Check sheet for the modelled part. Datum: model origin and axes. Units: mm. Face numbers are marked on the shaded views. A direction names the side the tool comes from. Give positions to 0.01 mm unless a question says otherwise; leave off trailing zeros. Order: outer loops, then holes, each group sorted by start corner. A loop starts at its lowest first (then second) coordinate and runs counter-clockwise, first axis right, second up.
from build123d import *

# Parameters (mm, degrees)
SKETCH2_R           = 6.5
BOSS_EXTRUDE1_DEPTH = 7


with BuildPart() as part:
    # Sketch1 → Revolve1 (revolve)
    with BuildSketch(Plane.XY):
        with BuildLine():
            Line((0, 6.5), (0, 10.5))
            Line((0, 10.5), (22.5, 10.5))
            Line((22.5, 10.5), (22.5, 7.5))
            Line((22.5, 7.5), (10.5, 7.5))
            ThreePointArc((10.5, 7.5), (10.146446609, 7.353553391), (10, 7))
            Line((10, 7), (10, 6.5))
            Line((10, 6.5), (0, 6.5))
        make_face()
    revolve(axis=Axis((0, 0, 0), (1, 0, 0)))

    # Sketch2 → Boss-Extrude1 (add)
    with BuildSketch(Plane.ZY):
        Polygon((0, 13.279056191), (-11.5, 6.639528096), (-11.5, -6.639528096), (0, -13.279056191), (11.5, -6.639528096), (11.5, 6.639528096), align=None)
        Circle(SKETCH2_R, mode=Mode.SUBTRACT)
    extrude(amount=-BOSS_EXTRUDE1_DEPTH)

    # Cut-Sweep1: sweep along a path in Sketch6
    with BuildLine(Plane.ZY) as cut_sweep1_path:
        CenterArc((0, 0), 11.5, 0, 360)
    # Sketch5 → Cut-Sweep1 (sweep, cut)
    with BuildSketch(Plane.XY):
        with BuildLine():
            Line((0.6, 13.279056191), (0, 13.279056191))
            Line((0, 13.279056191), (0, 11))
            ThreePointArc((0, 11), (0.152512755, 12.178356602), (0.6, 13.279056191))
        make_face()
    sweep(path=cut_sweep1_path.line, mode=Mode.SUBTRACT)


solid = part.part
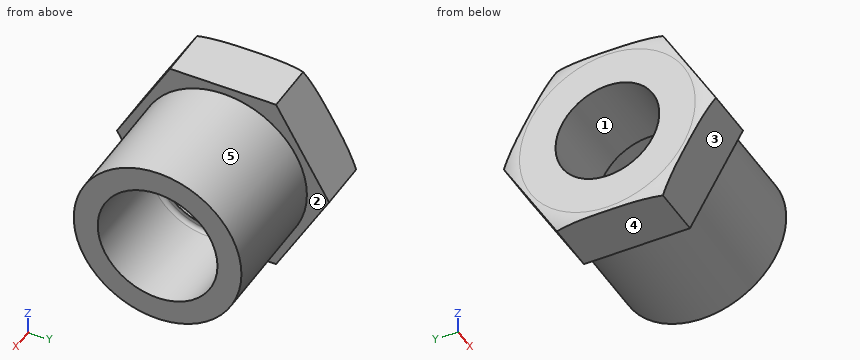
1) Set-up check for the marked faces 4 and 5: record each of +Z, -Z, +X, -X, +Y, -Y from which the full face is reachable in a straight line by a thin tool's end or side.
Recorded:
face 4: -Z, +X, -X, +Y, -Y
face 5: +X
2) Section check C-C, the plane x = 17.5. Record the cut outline in (y, z).
Recorded:
outline: circle Ø21 at (0, 0); hole circle Ø15 at (0, 0)
3) Section check A-A, the plane y = 0. Record the cut outline in (x, z).
Recorded:
outline: (0, -11) arc R4.63 ccw to (0.03, -11.5) - (7, -11.5) - (7, -10.5) - (22.5, -10.5) - (22.5, -7.5) - (10.5, -7.5) arc R0.5 cw to (10, -7) - (10, -6.5) - (0, -6.5) - close; (0, 6.5) - (10, 6.5) - (10, 7) arc R0.5 cw to (10.5, 7.5) - (22.5, 7.5) - (22.5, 10.5) - (7, 10.5) - (7, 11.5) - (0.03, 11.5) arc R4.63 ccw to (0, 11) - close
4) Section check B-B, the plane x = 5. Record the cut outline in (y, z).
Recorded:
outline: (-13.28, 0) - (-6.64, -11.5) - (6.64, -11.5) - (13.28, 0) - (6.64, 11.5) - (-6.64, 11.5) - close; hole circle Ø13 at (0, 0)
5) Depth check by flat-ended pin: pin 1 Ø1.5 at (x, z) = (6.5, -6) entering from -Y; pin 2 Ø10 at (x, z) = (16.5, 8) entering from -Y; pin 3 Ø1 at (x, y) = (20, -10) entering from -Z. Enter the tip coordinate at first touch or a pass-through.
Recorded:
pin 1: stops at y = -10.25
pin 2: stops at y = -10.06
pin 3: stops at z = -4.47
6) Draft check along Z on the marked faces 1, 2 and 3. Enter one of: +Z half, -Z half, draft (parallel to the pull), parting line (faces both ways), or undercut.
Recorded:
face 1: undercut
face 2: draft
face 3: -Z half
7) Material ranges on L1, parallel to Z at x = 4.75, y = 0; L2, parallel to Z at x = 16.75, y = 0; L3, parallel to Y at x = 9.25, z = 1.75, recorded low to high.
Recorded:
L1: z = -11.5 to -6.5, 6.5 to 11.5
L2: z = -10.5 to -7.5, 7.5 to 10.5
L3: y = -10.35 to -6.26, 6.26 to 10.35
